Work out the finished part from the listing and answer in its coordinate system (mm). Coordinates: 2 decimals unless noted, no trailing zeros. Order: outer loops, then holes, each group sorted by start corner. A loop starts at its lowest first (then second) coordinate and runs counter-clockwise, first axis right, second up. Notation, with made-up numbers: (22.25, 4) -> (28.25, 4) arc R13 ccw to (28.25, 21) -> close; hole circle Ø3 at (-29.5, -14.75). An arc over 180 degrees is marked (long way). Answer as CSV lines item,"result". Start each with the question number.
Item 1: Section A-A (x = 0) is taken. Write down the section's boundary in (y, z), then the cut area to 3 significant figures.
Item 2: Straight lines are drawn through the part: L1, parallel to X at y = -13, z = -14.5; L2, parallel to X at y = -11, z = 27.5; L3, parallel to X at y = -12.5, z = -1. For each, find the intervals that lie inside material, in ascending order.
Item 3: Section B-B (z = 0) is taken. Write down the section's boundary in (x, y), then the cut area to 3 significant figures.
Item 4: Section C-C (y = -5) is taken. Write down the section's boundary in (x, z).
Item 5: For a pull along X with two mould halves and no side action, classify faces 1 (the face through (113.607, -12.325, -12.75)), 2 (the face through (-62.106, -12, -2)), 3 (the face through (34, -12, -64.315)) as pulls with the +X half, pulls with the -X half, needs draft (parallel to the pull), parting line crosses it, or undercut.
```python
from build123d import *

# Parameters (mm, degrees)
F0_W     = 194.955856
F0_H     = 126.944736
F0_R     = 6.365504
F0_R_2   = 48.999093
F0_R_3   = 6.600609
F1_DEPTH = 25


with BuildPart() as f1:
    # F0 (on Front) → F1 (new body)
    with BuildSketch(Plane.XZ):
        with Locations((35.371989, -0.842303)):
            Rectangle(F0_W, F0_H)
        with Locations((107.535303, -14.661582)):
            Circle(F0_R, mode=Mode.SUBTRACT)
        Circle(F0_R_2, mode=Mode.SUBTRACT)
        with Locations((104.284093, 23.773747)):
            Circle(F0_R_3, mode=Mode.SUBTRACT)
    extrude(amount=F1_DEPTH)


solid = f1.part
```
Checked values:
1,outline,"(-25, -64.31) -> (0, -64.31) -> (0, -49) -> (-25, -49) -> close; (-25, 49) -> (0, 49) -> (0, 62.63) -> (-25, 62.63) -> close"
1,area,"724 mm^2"
2,L1,"x = -62.11 to -46.8, 46.8 to 101.17, 113.9 to 132.85"
2,L2,"x = -62.11 to -40.55, 40.55 to 98.84, 109.73 to 132.85"
2,L3,"x = -62.11 to -48.99, 48.99 to 132.85"
3,outline,"(-62.11, -25) -> (-49, -25) -> (-49, 0) -> (-62.11, 0) -> close; (49, -25) -> (132.85, -25) -> (132.85, 0) -> (49, 0) -> close"
3,area,"2,420 mm^2"
4,outline,"(-62.11, -64.31) -> (132.85, -64.31) -> (132.85, 62.63) -> (-62.11, 62.63) -> close; hole circle Ø98 at (0, 0); hole circle Ø13.2 at (104.28, 23.77); hole circle Ø12.73 at (107.54, -14.66)"
5,face 1,"undercut"
5,face 2,"pulls with the -X half"
5,face 3,"needs draft"
